CAD build for the part. Positions are in the model's coordinates, mm. Round coordinates to 2 decimals unless told otherwise and drop trailing zeros. Write each loop counter-clockwise with the first axis right and the second up, starting at its lowest first coordinate (ties: lowest second). Pieces come first, ordered by that corner, then holes. Notation, with made-up numbers: (-1, 5) - (6, 5) arc R10 cw to (6, 9) - close; hole circle Ø5 at (-20, 7.5). An arc over 180 degrees is marked (long way). Use one line per item in the form item = value. Start each with the question number.
Item 1: Band-saw the part on D-D, the plane z = -60. List the corners of the cut face in (x, y).
Item 2: Pin check, flat tips, straight feed: pin 1 (4 mm diameter, centred on x = 261.5, z = -108.5, fed in from -Y); pin 2 (1.5 mm diameter, centred on x = 266.5, y = 1.5, fed in from +Z). Stop position of each tip, or through.
Item 3: Band-saw the part on B-B, the plane z = 16. List the corners of the cut face in (x, y), and give its area (3 significant figures).
Item 4: Band-saw the part on A-A, the plane y = 2.9. Give the number of separate pieces and of enclosed holes in the cut face, and give its area (3 significant figures).
Item 5: Band-saw the part on C-C, the plane x = 225. List the corners of the cut face in (y, z), and give its area (3 significant figures).
Item 6: Drill centre lines: L1, parallel to X at y = 2.1, z = -60; L2, parallel to X at y = 3.85, z = 8; L3, parallel to Z at x = 423, y = 3.4. Where is each one in solid material? Low to high.
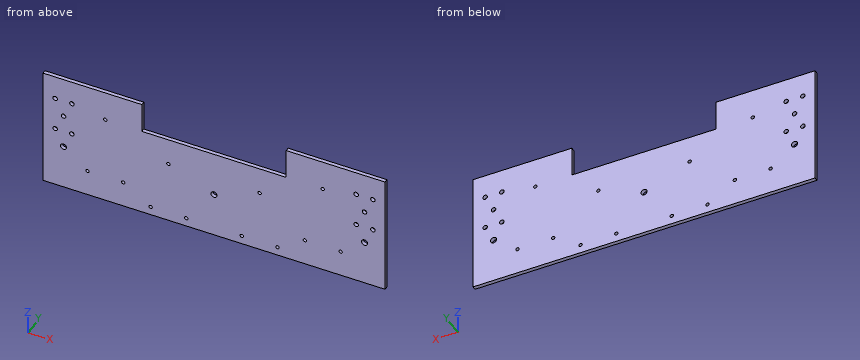
from build123d import *

# Parameters (mm, degrees)
SKETCH_1_W          = 450
SKETCH_1_H          = 120
EXTRUDE_1_DEPTH     = 5
SKETCH_2_R          = 4
CUT_EXTRUDE_1_DEPTH = 466.752079974
SKETCH_3_R          = 2.25
CUT_EXTRUDE_2_DEPTH = 466.752079974
SKETCH_4_W          = 130
SKETCH_4_H          = 40
EXTRUDE_2_DEPTH     = 5
SKETCH_5_R          = 2.25
CUT_EXTRUDE_3_DEPTH = 466.752079974
SKETCH_7_R          = 3
CUT_EXTRUDE_4_DEPTH = 466.752079974


with BuildPart() as part:
    # 草图1 → 凸台-拉伸1 (new body)
    with BuildSketch(Plane(origin=(0, 0, 0), x_dir=(1, 0, 0), z_dir=(0, 1, 0))):
        with Locations((225, 60)):
            Rectangle(SKETCH_1_W, SKETCH_1_H)
    extrude(amount=EXTRUDE_1_DEPTH)

    # 草图2 → 切除-拉伸1 (cut, through all)
    with BuildSketch(Plane(origin=(0, 5, 0), x_dir=(1, 0, 0), z_dir=(0, 1, 0))):
        with Locations(Location((225, 60, 0), (0, 0, 270))):
            Circle(SKETCH_2_R)
        with Locations(Location((27, 60, 0), (0, 0, 270))):
            Circle(SKETCH_2_R)
        with Locations(Location((423, 60, 0), (0, 0, 90))):
            Circle(SKETCH_2_R)
    extrude(amount=-CUT_EXTRUDE_1_DEPTH, mode=Mode.SUBTRACT)

    # 草图3 → 切除-拉伸2 (cut, through all)
    with BuildSketch(Plane(origin=(0, 5, 0), x_dir=(1, 0, 0), z_dir=(0, 1, 0))):
        with Locations(Location((165, 36, 0), (0, 0, 270))):
            Circle(SKETCH_3_R)
        with Locations(Location((141.5, 108.5, 0), (0, 0, 270))):
            Circle(SKETCH_3_R)
        with Locations(Location((188.5, 108.5, 0), (0, 0, 90))):
            Circle(SKETCH_3_R)
        with Locations(Location((285, 36, 0), (0, 0, 90))):
            Circle(SKETCH_3_R)
        with Locations(Location((261.5, 108.5, 0), (0, 0, 270))):
            Circle(SKETCH_3_R)
        with Locations(Location((308.5, 108.5, 0), (0, 0, 90))):
            Circle(SKETCH_3_R)
    extrude(amount=-CUT_EXTRUDE_2_DEPTH, mode=Mode.SUBTRACT)

    # 草图4 → 凸台-拉伸2 (add)
    with BuildSketch(Plane(origin=(0, 5, 0), x_dir=(1, 0, 0), z_dir=(0, 1, 0))):
        with Locations((65, -20)):
            Rectangle(SKETCH_4_W, SKETCH_4_H)
        with Locations((385, -20)):
            Rectangle(SKETCH_4_W, SKETCH_4_H)
    extrude(amount=-EXTRUDE_2_DEPTH)

    # 草图5 → 切除-拉伸3 (cut, through all)
    with BuildSketch(Plane(origin=(0, 5, 0), x_dir=(1, 0, 0), z_dir=(0, 1, 0))):
        with Locations(Location((82, 0, 0), (0, 0, 270))):
            Circle(SKETCH_5_R)
        with Locations(Location((58.5, 85, 0), (0, 0, 270))):
            Circle(SKETCH_5_R)
        with Locations(Location((105.5, 85, 0), (0, 0, 90))):
            Circle(SKETCH_5_R)
        with Locations(Location((368, 0, 0), (0, 0, 90))):
            Circle(SKETCH_5_R)
        with Locations(Location((344.5, 85, 0), (0, 0, 270))):
            Circle(SKETCH_5_R)
        with Locations(Location((391.5, 85, 0), (0, 0, 90))):
            Circle(SKETCH_5_R)
    extrude(amount=-CUT_EXTRUDE_3_DEPTH, mode=Mode.SUBTRACT)

    # 草图7 → 切除-拉伸4 (cut, through all)
    with BuildSketch(Plane(origin=(0, 5, 0), x_dir=(1, 0, 0), z_dir=(0, 1, 0))):
        with Locations(Location((38, 37, 0), (0, 0, 270))):
            Circle(SKETCH_7_R)
        with Locations(Location((16, 37, 0), (0, 0, 90))):
            Circle(SKETCH_7_R)
        with Locations(Location((16, -8, 0), (0, 0, 270))):
            Circle(SKETCH_7_R)
        with Locations(Location((38, -8, 0), (0, 0, 90))):
            Circle(SKETCH_7_R)
        with Locations(Location((27, 14.5, 0), (0, 0, 270))):
            Circle(SKETCH_7_R)
        with Locations(Location((412, 37, 0), (0, 0, 90))):
            Circle(SKETCH_7_R)
        with Locations(Location((434, 37, 0), (0, 0, 270))):
            Circle(SKETCH_7_R)
        with Locations(Location((434, -8, 0), (0, 0, 90))):
            Circle(SKETCH_7_R)
        with Locations(Location((423, 14.5, 0), (0, 0, 90))):
            Circle(SKETCH_7_R)
        with Locations(Location((412, -8, 0), (0, 0, 270))):
            Circle(SKETCH_7_R)
    extrude(amount=-CUT_EXTRUDE_4_DEPTH, mode=Mode.SUBTRACT)


solid = part.part
Determined:
q1.outline = (0, 0) - (23, 0) - (23, 5) - (0, 5) - close; (31, 0) - (221, 0) - (221, 5) - (31, 5) - close; (229, 0) - (419, 0) - (419, 5) - (229, 5) - close; (427, 0) - (450, 0) - (450, 5) - (427, 5) - close
q2.pin_1 = through
q2.pin_2 = 0
q3.outline = (0, 0) - (130, 0) - (130, 5) - (0, 5) - close; (320, 0) - (450, 0) - (450, 5) - (320, 5) - close
q3.area = 1,300 mm²
q4.separate_pieces = 1
q4.enclosed_holes = 25
q4.area = 63,800 mm²
q5.outline = (0, -120) - (5, -120) - (5, -64) - (0, -64) - close; (0, -56) - (5, -56) - (5, 0) - (0, 0) - close
q5.area = 560 mm²
q6.L1 = 0 to 23, 31 to 221, 229 to 419, 427 to 450
q6.L2 = 0 to 13, 19 to 35, 41 to 130, 320 to 409, 415 to 431, 437 to 450
q6.L3 = -120 to -64, -56 to -17.5, -11.5 to 40
